Check sheet for the modelled part. Datum: model origin and axes. Units: mm. Round coordinates to 2 decimals unless told otherwise and drop trailing zeros. Order: outer loops, then holes, each group sorted by start corner. A loop starts at its lowest first (then second) coordinate and runs counter-clockwise, first axis right, second up.
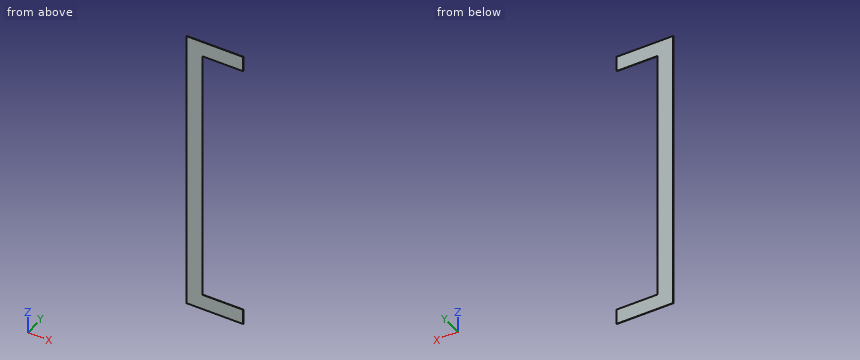
Autodesk Inventor part; units mm, degrees
ref_plane "YZ Plane" through (0, 0, 0) normal (1, 0, 0) x (0, 1, 0)
ref_plane "XZ Plane" through (0, 0, 0) normal (0, 1, 0) x (-1, 0, 0)
ref_plane "XY Plane" through (0, 0, 0) normal (0, 0, 1) x (1, 0, 0)
sketch "スケッチ1" plane through (0, 0, 0) normal (0, 1, 0) x (-1, 0, 0)
  line L0 (-145, -750) -> (145, -750)
  line L1 (145, -750) -> (145, 750)
  line L2 (145, 750) -> (-145, 750)
  line L3 (-145, 750) -> (-145, -750)
  line L4 (-145, -750) -> (145, 750) construction
  line L5 (145, -750) -> (-145, 750) construction
  point P0 (0, 0)
  dimension "d0" = 1500
  dimension "d1" = 290
extrude "押し出し1" add sketch "スケッチ1" along normal blind 2
sketch "スケッチ2" plane through (0, 2, 0) normal (0, 1, 0) x (1, 0, 0)
  line L0 (355, 670) -> (-65, 670)
  line L1 (-65, 670) -> (-65, -670)
  line L2 (-65, -670) -> (355, -670)
  line L3 (355, -670) -> (355, 670)
  line L4 (145, -750) -> (145, 750)
  line L5 (355, 670) -> (-65, -670) construction
  line L6 (-65, 670) -> (355, -670) construction
  line L7 (-145, -750) -> (145, -750)
  line L8 (-145, 750) -> (-145, -750)
  point P0 (0, 0)
  point P1 (145, 0)
  point P2 (145, -670)
  point P3 (145, 670)
  dimension "d4" = 80
  dimension "d5" = 80
extrude "押し出し2" cut sketch "スケッチ2" against normal blind 10 contours L4 L2 L1 L0
properties part number "Panel_E" material "アルミニウム 6061"
Item 1: Scan lines: line 1 along Z through (x, y) = (30, 1.15); line 2 along X through (y, z) = (1, -241.5). Record each from-to range of solid material in increasing order.
Answer:
line 1: z = -750 to -670, 670 to 750
line 2: x = -145 to -65
Item 2: Sectioned sample at C-C (z = 578). Record the cut outline in (x, y).
Answer:
outline: (-145, 0) - (-65, 0) - (-65, 2) - (-145, 2) - close
Item 3: Sectioned sample at B-B (y = 0.85). Record the cut outline in (x, z).
Answer:
outline: (-145, -750) - (145, -750) - (145, -670) - (-65, -670) - (-65, 670) - (145, 670) - (145, 750) - (-145, 750) - close
Item 4: Sectioned sample at A-A (x = 35.5). Record the cut outline in (y, z), and give its area (3 significant figures).
Answer:
outline: (0, -750) - (2, -750) - (2, -670) - (0, -670) - close; (0, 670) - (2, 670) - (2, 750) - (0, 750) - close
area: 320 mm2
Item 5: Go/stop test with a flat-tipped pin: P1, Ø10, axis at x = -108, z = 548, coming from the -Y side. Record where the tip stops, or that it passes through.
Answer:
P1: stops at y = 0
